Geometry: final body of the model. Coordinates: model frame, mm. A direction names the side the tool comes from. Round coordinates to 2 decimals unless told otherwise and drop trailing zeros. Write each loop counter-clockwise with the first axis right and the second up, starting at its lowest first coordinate (ties: lowest second). Pieces come first, ordered by that corner, then holes. Notation, with made-up numbers: M 69,28.5 L 128,28.5 A5 ccw 128,35.5 Z; hole C -36,42.5 d5. An arc over 180 degrees is marked long. Answer as CSV lines item,"result". Start each with the question number.
Q1. Ray query, probe 1 along Z at (x, y) = (54.5, 42.5); probe 2 along Y at (x, z) = (-15.5, 8.5). Return the intervals inside material, ascending.
Q2. Section query C-C on y = -78.5. Output: boundary loops of the cut face in (x, z), and give its area (3 significant figures).
Q3. Reachability of faces 1 (the flat face through (0, -90, 15)), 2 (the flat face through (-20, -95, 15)), 3 (the flat face through (20, -95, 15)) from +Z, -Z, +X, -X, +Y, -Y: full face, straight path, thin tool, end or side. Return the list, or none.
Q4. First-contact query: pin 1 (6 mm diameter, centred on x = -0.5, z = 12, fed in from +Y); pin 2 (6 mm diameter, centred on x = -59.5, y = 6.5, fed in from +Z); pin 3 (6 mm diameter, centred on x = -87, y = 8, fed in from -Z); pin 4 (3 mm diameter, centred on y = -97, z = 17.5, fed in from +X). Flat tips, straight axial feed; report the tip coordinate or a pass-through.
Q5. Section query B-B on z = 9.25. Output: boundary loops of the cut face in (x, y).
Q6. Section query A-A on x = 5.5. Output: boundary loops of the cut face in (y, z), and give its area (3 significant figures).
```python
from build123d import *

# Parameters (mm, degrees)
SKETCH1_W           = 300
SKETCH1_H           = 200
BOSS_EXTRUDE1_DEPTH = 5
SKETCH3_W           = 20
SKETCH3_H           = 20
SKETCH3_H_2         = 40
CUT_EXTRUDE1_DEPTH  = 5
SKETCH4_W           = 20
SKETCH4_H           = 140
CUT_EXTRUDE2_DEPTH  = 10
SKETCH6_W           = 40
SKETCH6_H           = 25
BOSS_EXTRUDE3_DEPTH = 10


with BuildPart() as part:
    # Sketch1 → Boss-Extrude1 (new body)
    with BuildSketch(Plane.XY):
        Rectangle(SKETCH1_W, SKETCH1_H)
    extrude(amount=BOSS_EXTRUDE1_DEPTH)

    # Sketch3 → Cut-Extrude1 (cut)
    with BuildSketch(Plane.XY.offset(5)):
        with Locations((-140, -90)):
            Rectangle(SKETCH3_W, SKETCH3_H)
        with Locations((-140, 80)):
            Rectangle(SKETCH3_W, SKETCH3_H_2)
        with Locations((140, 80)):
            Rectangle(SKETCH3_W, SKETCH3_H_2)
        with Locations((140, -90)):
            Rectangle(SKETCH3_W, SKETCH3_H)
    extrude(amount=-CUT_EXTRUDE1_DEPTH, mode=Mode.SUBTRACT)

    # Sketch4 → Cut-Extrude2 (cut)
    with BuildSketch(Plane.XY.offset(5)):
        with Locations((-140, -10)):
            Rectangle(SKETCH4_W, SKETCH4_H)
        with Locations((140, -10)):
            Rectangle(SKETCH4_W, SKETCH4_H)
    extrude(amount=-CUT_EXTRUDE2_DEPTH, mode=Mode.SUBTRACT)

    # Sketch6 → Boss-Extrude3 (add)
    with BuildSketch(Plane.XZ.offset(100)):
        with Locations((0, 12.5)):
            Rectangle(SKETCH6_W, SKETCH6_H)
    extrude(amount=-BOSS_EXTRUDE3_DEPTH)


solid = part.part
```
Entries:
1,probe 1,"z = 0 to 5"
1,probe 2,"y = -100 to -90"
2,outline,"M -130,0 L 130,0 L 130,5 L -130,5 Z"
2,area,"1,300 mm^2"
3,face 1,"+Z, +X, -X, +Y"
3,face 2,"+Z, -X, +Y, -Y"
3,face 3,"+Z, +X, +Y, -Y"
4,pin 1,"stops at y = -90"
4,pin 2,"stops at z = 5"
4,pin 3,"stops at z = 0"
4,pin 4,"stops at x = 20"
5,outline,"M -20,-100 L 20,-100 L 20,-90 L -20,-90 Z"
6,outline,"M -100,0 L 100,0 L 100,5 L -90,5 L -90,25 L -100,25 Z"
6,area,"1,200 mm^2"
